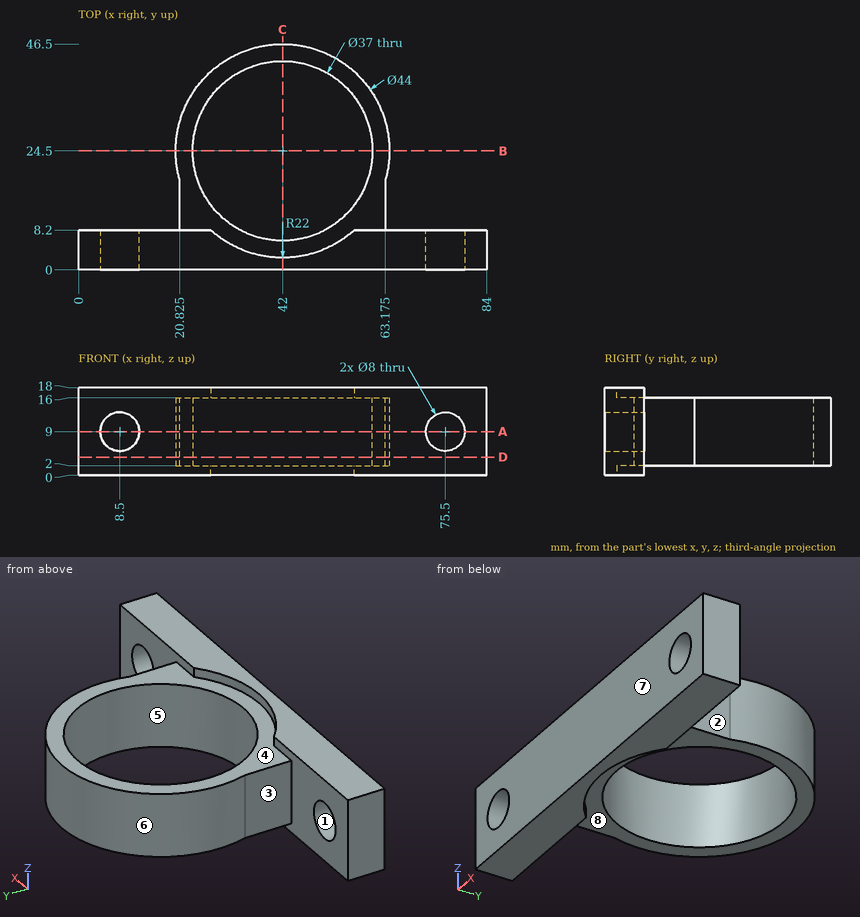
Design review of the part shown in the three views and the two pictorial views. Dimensions are in mm from the part's minimum x, y and z. A direction names the side the tool comes from. Give positions to 0.01 mm unless a question says otherwise; leave off trailing zeros. Loops run counter-clockwise (first coordinate to the right, second up) from the corner with the lowest first, then second, coordinate; pieces in that order, holes last. Notation, with made-up numbers: (64, 84) -> (110, 84) arc R13 ccw to (110, 97) -> close; hole circle Ø8 at (-20, -9.5). An arc over 180 degrees is marked (long way). Write each question's results on one line, items separated by ' | '.
Q1. Take a section at B-B, the plane y = 24.5. Write out the cut boundary in (x, z).
Reply:
outline: (20, 2) -> (23.5, 2) -> (23.5, 16) -> (20, 16) -> close; (60.5, 2) -> (64, 2) -> (64, 16) -> (60.5, 16) -> close
Q2. For pin 1 Ø1.5 at (y, z) = (13.5, 2) entering from -X (1 decimal); pin 2 Ø6.5 at (x, z) = (75.5, 9) entering from +Y; pin 3 Ø1 at (x, z) = (70, 14.5) entering from +Y; pin 4 Ø5 at (y, z) = (29, 11.5) entering from -X, all flat-tipped, find the tip position at first contact; note any pin that passes through.
Reply:
pin 1: stops at x = 20.8 | pin 2: passes through | pin 3: stops at y = 8.2 | pin 4: stops at x = 20.09
Q3. Machinability: for the marked faces 1, 2, 3, 4 and 5, which of the approach directions +Z, -Z, +X, -X, +Y, -Y give a long, thin tool a straight path to every point of the face, cutting with its end or side? Answer none if there is none.
Reply:
face 1: +Y, -Y | face 2: +Z, -Z, +X | face 3: +Z, -Z, -X | face 4: +Z, +Y | face 5: +Z, -Z
Q4. Wall thickness on L1, parallel to Z at x = 8.5, y = 2; L2, parallel to X at y = 24.5, z = 9; L3, parallel to X at y = 3.75, z = 9: over which ranges is each line inside the solid? List them lowest first.
Reply:
L1: z = 0 to 5, 13 to 18 | L2: x = 20 to 23.5, 60.5 to 64 | L3: x = 0 to 4.5, 12.5 to 71.5, 79.5 to 84
Q5. Take a section at A-A, the plane z = 9. Write out the cut boundary in (x, y) (1 decimal).
Reply:
outline: (0, 0) -> (4.5, 0) -> (4.5, 8.2) -> (0, 8.2) -> close; (12.5, 0) -> (71.5, 0) -> (71.5, 8.2) -> (63.2, 8.2) -> (63.2, 18.5) arc R22 ccw (long way) to (20.8, 18.5) -> (20.8, 8.2) -> (12.5, 8.2) -> close; (79.5, 0) -> (84, 0) -> (84, 8.2) -> (79.5, 8.2) -> close; hole circle Ø37 at (42, 24.5)
Q6. Take a section at C-C, the plane x = 42. Write out the cut boundary in (y, z), plus the area to 3 significant figures.
Reply:
outline: (0, 0) -> (2.5, 0) -> (2.5, 2) -> (6, 2) -> (6, 16) -> (2.5, 16) -> (2.5, 18) -> (0, 18) -> close; (43, 2) -> (46.5, 2) -> (46.5, 16) -> (43, 16) -> close | area: 143 mm²
Q7. The part is to be moulded in two halves that separate along Y. For the marked faces 6, 7 and 8, say which applies: +Y half, -Y half, draft (parallel to the pull), parting line (faces both ways), or undercut.
Reply:
face 6: undercut | face 7: -Y half | face 8: draft
Q8. Take a section at D-D, the plane z = 3.75. Write out the cut boundary in (x, y) (1 decimal).
Reply:
outline: (0, 0) -> (84, 0) -> (84, 8.2) -> (63.2, 8.2) -> (63.2, 18.5) arc R22 ccw (long way) to (20.8, 18.5) -> (20.8, 8.2) -> (0, 8.2) -> close; hole circle Ø37 at (42, 24.5)
